```python
from build123d import *

# Parameters (mm, degrees)
CROQUIS1_W              = 177.2
CROQUIS1_H              = 6.25
SALIENTE_EXTRUIR1_DEPTH = 3.125
CROQUIS4_R              = 1.5
CORTAR_EXTRUIR1_DEPTH   = 15
CROQUIS5_R              = 1.5
CORTAR_EXTRUIR3_DEPTH   = 368


with BuildPart() as part:
    # Croquis1 → Saliente-Extruir1 (new, symmetric)
    with BuildSketch(Plane(origin=(0, 0, 0), x_dir=(0, 0, -1), z_dir=(1, 0, 0))):
        Rectangle(CROQUIS1_W, CROQUIS1_H)
    extrude(amount=SALIENTE_EXTRUIR1_DEPTH, both=True)

    # Croquis4 → Cortar-Extruir1 (cut, symmetric)
    with BuildSketch(Plane(origin=(3.125, 0, 0), x_dir=(0, 0, -1), z_dir=(1, 0, 0))):
        with Locations(Location((85.475, 0, 0), (0, 0, 180))):
            Circle(CROQUIS4_R)
        with Locations(Location((77.975, 0, 0), (0, 0, 180))):
            Circle(CROQUIS4_R)
        with Locations(Location((-85.475, 0, 0), (0, 0, 180))):
            Circle(CROQUIS4_R)
        with Locations(Location((-77.975, 0, 0), (0, 0, 180))):
            Circle(CROQUIS4_R)
    extrude(amount=CORTAR_EXTRUIR1_DEPTH, both=True, mode=Mode.SUBTRACT)

    # Croquis5 → Cortar-Extruir3 (cut)
    with BuildSketch(Plane.XZ.offset(3.125)):
        with Locations(Location((0, -70.475, 0), (0, 0, 270))):
            Circle(CROQUIS5_R)
        with Locations(Location((0, 70.475, 0), (0, 0, 270))):
            Circle(CROQUIS5_R)
    extrude(amount=-CORTAR_EXTRUIR3_DEPTH, mode=Mode.SUBTRACT)


solid = part.part
```
Part model, mm, in its own coordinate system. Give positions to 0.01 mm unless a question says otherwise; leave off trailing zeros. Write each loop counter-clockwise with the first axis right and the second up, starting at its lowest first coordinate (ties: lowest second). Pieces come first, ordered by that corner, then holes. Notation, with made-up numbers: M -32,6.5 L 19,6.5 A32 cw 19,34.5 Z; hole C -23,-18.75 d10. An arc over 180 degrees is marked long. Use CSV: the item, a comma, the result in double quotes.
Item 1: Pull direction X, two halves, no side cores. Call faces 1 (the face through (0, 3.125, 1)), 2 (the face through (3.125, 0, 1)), 3 (the face through (0.451, -0.044, -71.906)): +X half, -X half, draft (parallel to the pull), parting line (faces both ways), or undercut.
Taken from the geometry:
face 1,"draft"
face 2,"+X half"
face 3,"undercut"
Item 2: Drill centre lines: probe 1 along Z at (x, y) = (3, 1.25); probe 2 along Z at (x, y) = (0.5, 2.25); probe 3 along Z at (x, y) = (-3, 0.5). Where is each one in solid material? Low to high.
Taken from the geometry:
probe 1,"z = -88.6 to -86.3, -84.65 to -78.8, -77.15 to 77.15, 78.8 to 84.65, 86.3 to 88.6"
probe 2,"z = -88.6 to -71.89, -69.06 to 69.06, 71.89 to 88.6"
probe 3,"z = -88.6 to -86.89, -84.06 to -79.39, -76.56 to 76.56, 79.39 to 84.06, 86.89 to 88.6"
Item 3: Slice it at B-B on x = 0. Write the cut outline in (y, z) (3 decimals).
Taken from the geometry:
outline,"M -3.125,-88.6 L 3.125,-88.6 L 3.125,-71.975 L -3.125,-71.975 Z; M -3.125,-68.975 L 3.125,-68.975 L 3.125,68.975 L -3.125,68.975 Z; M -3.125,71.975 L 3.125,71.975 L 3.125,88.6 L -3.125,88.6 Z; hole C 0,-85.475 d3; hole C 0,-77.975 d3; hole C 0,77.975 d3; hole C 0,85.475 d3"
Item 4: Slice it at A-A on y = 0. Write the cut outline in (x, z) (3 decimals).
Taken from the geometry:
outline,"M -3.125,-88.6 L 3.125,-88.6 L 3.125,-86.975 L -3.125,-86.975 Z; M -3.125,-83.975 L 3.125,-83.975 L 3.125,-79.475 L -3.125,-79.475 Z; M -3.125,-76.475 L 3.125,-76.475 L 3.125,76.475 L -3.125,76.475 Z; M -3.125,79.475 L 3.125,79.475 L 3.125,83.975 L -3.125,83.975 Z; M -3.125,86.975 L 3.125,86.975 L 3.125,88.6 L -3.125,88.6 Z; hole C 0,-70.475 d3; hole C 0,70.475 d3"
